The model under review builds one solid part; all positions refer to its coordinate system, in mm. Give positions to 0.01 mm unless a question says otherwise; leave off trailing zeros. Write each loop counter-clockwise with the first axis right and the second up, starting at its lowest first coordinate (ties: lowest second). Pieces come first, ordered by that corner, then holes. Notation, with made-up numbers: (64.25, 1.5) - (88.25, 1.5) arc R26 cw to (88.25, 36.5) - close; hole circle Ø2 at (87.5, 73). An arc over 180 degrees is marked (long way). Write item = value, one per line.
```python
from build123d import *

# Parameters (mm, degrees)
SKETCH1_R           = 96
SKETCH1_R_2         = 60
BOSS_EXTRUDE1_DEPTH = 2
SKETCH2_R           = 4.25
CUT_EXTRUDE1_DEPTH  = 136.823414771
CIRPATTERN1_COUNT   = 20
CHAMFER1_SIZE       = 3
CHAMFER1_SIZE2      = 1.732050808


with BuildPart() as part:
    # Sketch1 → Boss-Extrude1 (new, symmetric)
    with BuildSketch(Plane(origin=(0, 0, 0), x_dir=(0, 0, -1), z_dir=(1, 0, 0))):
        Circle(SKETCH1_R)
        Circle(SKETCH1_R_2, mode=Mode.SUBTRACT)
    extrude(amount=BOSS_EXTRUDE1_DEPTH, both=True)

    # Sketch2 → Cut-Extrude1 (cut, through all)
    with BuildSketch(Plane(origin=(2, 0, 0), x_dir=(0, 0, -1), z_dir=(1, 0, 0))):
        with Locations((0, 70)):
            Circle(SKETCH2_R)
        with BuildLine():
            Line((10.490232723, 55.175649906), (-0.23164627, 55.175649906))
            Line((-0.23164627, 55.175649906), (-10.490232723, 55.175649906))
            ThreePointArc((-10.490232723, 55.175649906), (-13.137614633, 61.283337309), (-6.588851569, 62.477564557))
            ThreePointArc((-6.588851569, 62.477564557), (0, 60), (6.588851569, 62.477564557))
            ThreePointArc((6.588851569, 62.477564557), (13.137614633, 61.283337309), (10.490232723, 55.175649906))
        make_face()
    cut_extrude1 = extrude(amount=-CUT_EXTRUDE1_DEPTH, mode=Mode.SUBTRACT)

    # CirPattern1: Cut-Extrude1 ×20 about axis
    cirpattern1_axis = Axis((0, 0, 0), (1, 0, 0))
    for i in range(1, CIRPATTERN1_COUNT):
        add(cut_extrude1.rotate(cirpattern1_axis, i * 360 / CIRPATTERN1_COUNT), mode=Mode.SUBTRACT)

    # Chamfer1
    chamfer1_edges = [part.edges().sort_by_distance(p)[0] for p in [
        (-2, 0, 96),
    ]]
    chamfer1_side = [part.faces().sort_by_distance(p)[0] for p in [
        (-2, 0, 93.28470996),
    ]]
    chamfer(chamfer1_edges, length=CHAMFER1_SIZE, length2=CHAMFER1_SIZE2, reference=chamfer1_side[0])


solid = part.part
```
1. Insertion check: P1, Ø7, axis at y = 21.63, z = -66.57, coming from the +X side; P2, Ø1.5, axis at x = -0.5, z = -75, coming from the -Y side; P3, Ø1, axis at y = 60.5, z = -75, coming from the -X side. Each pin has a flat end and moves straight along its axis. Give the tip position at first contact, or say it passes through.
Findings below:
P1 = through
P2 = -60.81
P3 = -0.35
2. Take a section at B-B on x = 0.7. Count the separate pieces of the cut face and the enclosed holes in it, and give its area (3 significant figures).
Findings below:
separate_pieces = 1
enclosed_holes = 21
area = 15,800 mm²
3. For line 1 (Y direction, x = -0.65, z = 21); line 2 (Y direction, x = -0.8, z = 64); line 3 (Y direction, x = 1.35, z = -22), list the stretches that pass through material, from the lowest coordinate up. Write a range as from..to.
Findings below:
line_1 = -93..-70.78, -62.37..-56.59, 56.59..62.37, 70.78..93
line_2 = -70.31..-25.01, -18.25..18.25, 25.01..70.31
line_3 = -93.45..-70.81, -62.34..-56.58, 56.58..62.34, 70.81..93.45
4. Take a section at A-A on y = 0. Give the boundary of the cut face in (x, z).
Findings below:
outline = (-2, -93) - (-0.27, -96) - (2, -96) - (2, -74.25) - (-2, -74.25) - close; (-2, -65.75) - (2, -65.75) - (2, -60) - (-2, -60) - close; (-2, 60) - (2, 60) - (2, 65.75) - (-2, 65.75) - close; (-2, 74.25) - (2, 74.25) - (2, 96) - (-0.27, 96) - (-2, 93) - close
5. Draft analysis for pull direction Y (two halves, no side actions). For faces 1 (the cylindrical face through (0.882, 4.221, 95.907)), 2 (the cylindrical face through (0.03, 35.19, 48.6)), state which applies: +Y half, -Y half, draft (parallel to the pull), parting line (faces both ways), or undercut.
Findings below:
face_1 = parting line
face_2 = undercut
